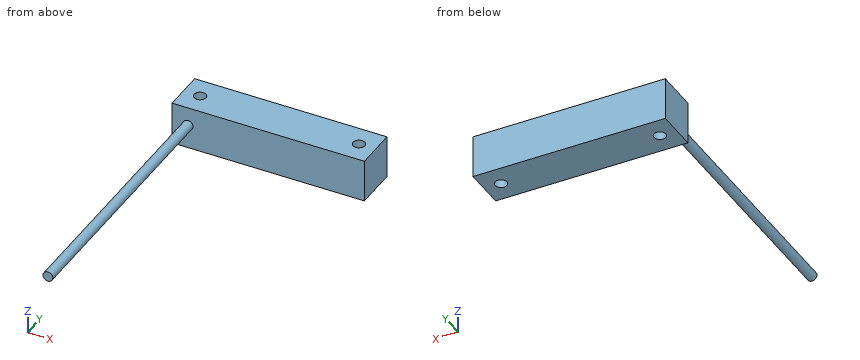
from build123d import *

# Parameters (mm, degrees)
F0_W     = 45.72
F0_H     = 10.16
F1_DEPTH = 10.16
F2_R     = 1.409591
F3_DEPTH = 25.4
F4_R     = 1.168764
F5_DEPTH = 62.992


with BuildPart() as f1:
    # F0 (on Top) → F1 (new body)
    with BuildSketch(Plane.XY):
        Rectangle(F0_W, F0_H)
    extrude(amount=F1_DEPTH)

    # F2 (on face) → F3 (cut)
    with BuildSketch(Plane.XY.offset(10.16)):
        with Locations((-18.874988, 0)):
            Circle(F2_R)
        with Locations((18.874988, 0)):
            Circle(F2_R)
    extrude(amount=-F3_DEPTH, mode=Mode.SUBTRACT)

    # F4 (on face) → F5 (join)
    with BuildSketch(Plane.XZ.offset(5.08)):
        with Locations((-19.05, 5.778021)):
            Circle(F4_R)
    extrude(amount=F5_DEPTH)


solid = f1.part
For this review, take the finished solid that the model builds, in its own axes (mm). Round coordinates to 2 decimals unless told otherwise and drop trailing zeros. Order: outer loops, then holes, each group sorted by start corner. A loop starts at its lowest first (then second) coordinate and runs counter-clockwise, first axis right, second up. Notation, with made-up numbers: M 13.25,45.5 L 40.25,45.5 A10 ccw 40.25,57.5 Z; hole C -19.5,-10 d6. An arc over 180 degrees is marked long. Use a Markdown table: item, result. Add a question column.
Item 1: Add section B-B, the plane x = -19.05. Give the boundary of the cut face in (y, z).
Item 2: Add section A-A, the plane y = 0. Give the boundary of the cut face in (x, z).
Item 3: Add section D-D, the plane x = -7.5. Give the boundary of the cut face in (y, z).
Item 4: Insertion check: pin 1 (5 mm diameter, centred on x = -4, z = 9, fed in from -Y); pin 2 (4 mm diameter, centred on y = -42.5, z = 1.5, fed in from +X); pin 3 (2 mm diameter, centred on y = -13, z = 7.5, fed in from -X); pin 4 (3.5 mm diameter, centred on x = -18.87, y = 0, fed in from +Z). Each pin has a flat end and moves straight along its axis. Give the tip position at first contact, or say it passes through.
Item 5: Add section C-C, the plane z = 2.5. Give the boundary of the cut face in (x, y), then the cut area to 3 significant figures.
Item 6: To check wall thickness, follow line 1 along Y through (x, z) = (-8, 9.5); line 2 along Z through (x, y) = (-19.5, -8); line 3 along X through (y, z) = (-48, 5). State the ranges of each line that lie inside material, in increasing order.
Geometry results:
| question | item | result |
|---|---|---|
| 1 | outline | M -68.07,4.61 L -5.08,4.61 L -5.08,0 L -1.4,0 L -1.4,10.16 L -5.08,10.16 L -5.08,6.95 L -68.07,6.95 Z; M 1.4,0 L 5.08,0 L 5.08,10.16 L 1.4,10.16 Z |
| 2 | outline | M -22.86,0 L -20.28,0 L -20.28,10.16 L -22.86,10.16 Z; M -17.47,0 L 17.47,0 L 17.47,10.16 L -17.47,10.16 Z; M 20.28,0 L 22.86,0 L 22.86,10.16 L 20.28,10.16 Z |
| 3 | outline | M -5.08,0 L 5.08,0 L 5.08,10.16 L -5.08,10.16 Z |
| 4 | pin 1 | stops at y = -5.08 |
| 4 | pin 2 | passes through |
| 4 | pin 3 | stops at x = -19.97 |
| 4 | pin 4 | stops at z = 10.16 |
| 5 | outline | M -22.86,-5.08 L 22.86,-5.08 L 22.86,5.08 L -22.86,5.08 Z; hole C -18.87,0 d2.82; hole C 18.87,0 d2.82 |
| 5 | area | 452 mm² |
| 6 | line 1 | y = -5.08 to 5.08 |
| 6 | line 2 | z = 4.7 to 6.86 |
| 6 | line 3 | x = -19.92 to -18.18 |
